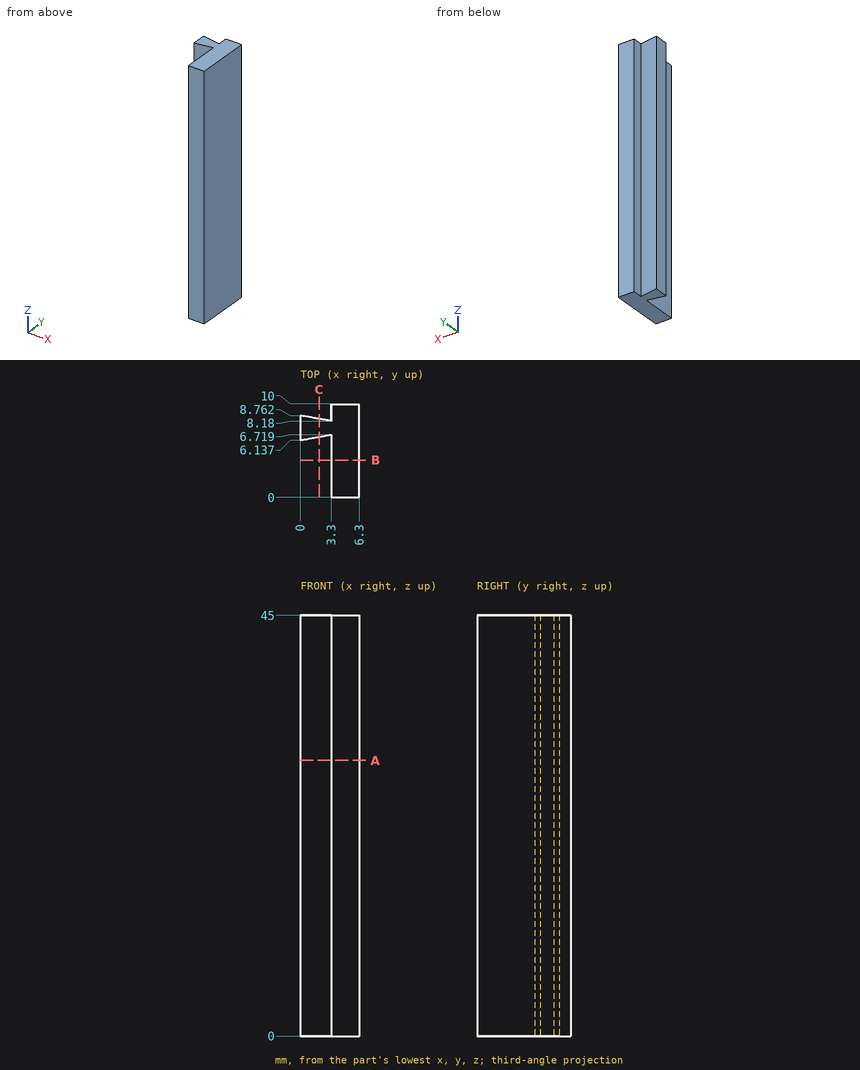
Design review of the part shown in the three views and the two pictorial views. Dimensions are in mm from the part's minimum x, y and z. Round coordinates to 2 decimals unless told otherwise and drop trailing zeros. Loops run counter-clockwise (first coordinate to the right, second up) from the corner with the lowest first, then second, coordinate; pieces in that order, holes last.
1) Wall thickness on line 1 along X through (y, z) = (1.25, 21); line 2 along Y through (x, z) = (3.25, 34); line 3 along Y through (x, z) = (1.5, 16.5): over which ranges is each line inside the solid? List them lowest first.
Values follow:
line 1: x = 3.3 to 6.3
line 2: y = 6.71 to 8.19
line 3: y = 6.4 to 8.5
2) Consider section C-C on x = 2. State the section outline as (y, z) points.
Values follow:
outline: (6.49, 0) - (8.41, 0) - (8.41, 45) - (6.49, 45) - close
3) Consider section B-B on y = 4. State the section outline as (x, z) points, then the cut area to 3 significant figures.
Values follow:
outline: (3.3, 0) - (6.3, 0) - (6.3, 45) - (3.3, 45) - close
area: 135 mm2
4) Consider section A-A on z = 29.5. State the section outline as (x, y) points.
Values follow:
outline: (0, 6.14) - (3.3, 6.72) - (3.3, 0) - (6.3, 0) - (6.3, 10) - (3.3, 10) - (3.3, 8.18) - (0, 8.76) - close
